Answer from the drawing. Dimensions are ordinates in mm from the lowest x, y and z of the part. Give positions to 0.01 mm unless a question says otherwise; leave off trailing zeros. Loops run counter-clockwise (first coordinate to the right, second up) from the corner with the lowest first, then second, coordinate; pieces in that order, holes last. Notation, with made-up numbers: (61, 19.5) - (111, 19.5) arc R16 ccw to (111, 37.5) - close; hole circle Ø1 at (-21, 73.25). An arc over 180 degrees is marked (long way). Put each result on its own line as item: value. Start each with the question number.
1. Consider L1, parallel to X at y = 72.5, z = 26; L2, parallel to Y at x = 302, z = 12 (1 decimal); L3, parallel to Z at x = 302, y = 101. Determine where each line is inside the solid, lowest interval first. Write a range as from..to.
2. A cutting plane is placed at A-A, the plane y = 54. Determine the outline of the cut face in (x, z).
3. A cutting plane is placed at B-B, the plane x = 165. Determine the outline of the cut face in (y, z).
4. Given pin 1 Ø6.5 at (y, z) = (101.6, 12.7) entering from -X; pin 2 Ø12 at (x, y) = (177, 30.5) entering from +Z, each flat-ended and moving along its own axis, determine where each tip first touches the part or whether it passes through.
5. For a pull along X with two mould halves and no side action, classify the marked faces 1, 2, 3 and 4 as released by +X, released by -X, zero draft, split by the parting line, or undercut.
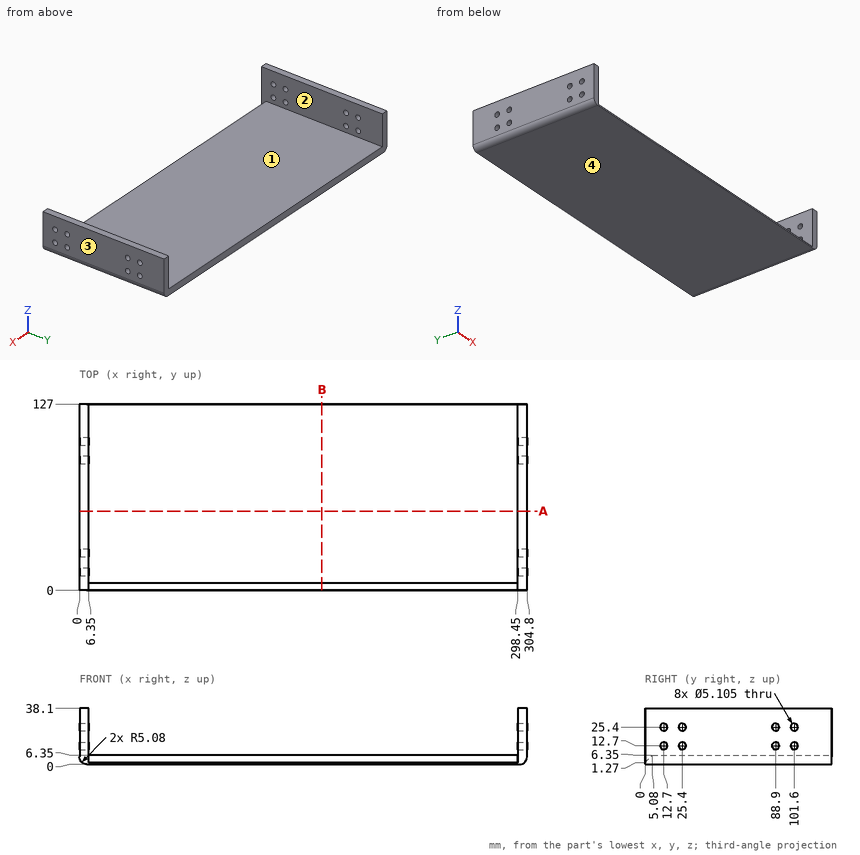
Return value:
1. L1: x = 0..6.35, 298.45..304.8
1. L2: y = 0..10.2, 15.2..22.9, 27.9..86.4, 91.4..99.1, 104.1..127
1. L3: z = 0.54..10.22, 15.18..22.92, 27.88..38.1
2. outline: (0, 5.08) arc R5.08 ccw to (5.08, 0) - (299.72, 0) arc R5.08 ccw to (304.8, 5.08) - (304.8, 38.1) - (298.45, 38.1) - (298.45, 6.35) - (6.35, 6.35) - (6.35, 38.1) - (0, 38.1) - close
3. outline: (0, 0) - (127, 0) - (127, 6.35) - (5.08, 6.35) - (0, 1.27) - close
4. pin 1: stops at x = 0
4. pin 2: stops at z = 6.35
5. face 1: undercut
5. face 2: undercut
5. face 3: released by +X
5. face 4: zero draft
